from build123d import *

# Parameters (mm, degrees)
CYLINDER012_R               = 2
CYLINDER012_DEPTH           = 15
CYLINDER012_PLACEMENT_ANGLE = 1
CYLINDER013_R               = 2
CYLINDER013_DEPTH           = 15
CYLINDER006_R               = 9.75
CYLINDER006_DEPTH           = 6
CYLINDER004_R               = 31.5
CYLINDER004_DEPTH           = 3


with BuildPart() as cylinder012:
    # Cylinder012 → Cylinder012 (new body)
    with BuildSketch(Plane.XY):
        Circle(CYLINDER012_R)
    extrude(amount=CYLINDER012_DEPTH)


with BuildPart() as cylinder012_1:
    # Cylinder012 placement: moved
    add(cylinder012.part.moved(Location((0, -15, -1))).rotate(Axis((0, -15, -1), (0, 0, 1)), CYLINDER012_PLACEMENT_ANGLE))


with BuildPart() as fusion004:
    # Cylinder013 → Cylinder013 (new body)
    with BuildSketch(Plane(origin=(0, 15, -1), x_dir=(1, 0, 0), z_dir=(0, 0, 1))):
        Circle(CYLINDER013_R)
    extrude(amount=CYLINDER013_DEPTH)

    # Fusion004: union Cylinder012
    add(cylinder012_1.part)


with BuildPart() as cylinder006:
    # Cylinder006 → Cylinder006 (new body)
    with BuildSketch(Plane.XY):
        Circle(CYLINDER006_R)
    extrude(amount=CYLINDER006_DEPTH)


with BuildPart() as end_flange001:
    # Cylinder004 → Cylinder004 (new body)
    with BuildSketch(Plane.XY):
        Circle(CYLINDER004_R)
    extrude(amount=CYLINDER004_DEPTH)

    # Cut001: cut Cylinder006
    add(cylinder006.part, mode=Mode.SUBTRACT)

    # Cut009: cut Fusion004
    add(fusion004.part, mode=Mode.SUBTRACT)


with BuildPart() as end_flange001_1:
    # Cut009 placement: moved
    add(end_flange001.part.moved(Location((65, 0, 0))))


solid = end_flange001_1.part
Check sheet for the modelled part. Datum: model origin and axes. Units: mm. Give positions to 0.01 mm unless a question says otherwise; leave off trailing zeros. Loops run counter-clockwise (first coordinate to the right, second up) from the corner with the lowest first, then second, coordinate; pieces in that order, holes last. Notation, with made-up numbers: M 23,80.25 L 66,80.25 A27 ccw 66,110.25 Z; hole C 66,78.5 d2. An arc over 180 degrees is marked long. Return JSON: item names as keys, results as strings. Group by question number.
1. Mould release check, pull along Y, two halves, no side actions. Record for faces 1 (the flat face through (71.6, 7.4, 0)), 2 (the cylindrical face through (65, -13, 1)), 3 (the cylindrical face through (41.783, 21.289, 1.479)): released by +Y, released by -Y, zero draft, split by the parting line, or undercut.
2. Cross-section at A-A on y = 0. Record the boundary of the cut face in (x, z).
3. Thickness scan on L1, parallel to Y at x = 65, z = 1.35; L2, parallel to X at y = -15, z = 1.55; L3, parallel to X at y = -13.5, z = 1.8. Record the ranges inside material, lowest first.
4. Cross-section at B-B on x = 65. Record the boundary of the cut face in (y, z), plus the area to 4 significant figures.
5. Go/stop test with flat-tipped pins: pin 1 (1.5 mm diameter, centred on y = -20, z = 2, fed in from +X); pin 2 (5 mm diameter, centred on x = 65, y = 15, fed in from -Z); pin 3 (11.5 mm diameter, centred on x = 65, y = 0, fed in from -Z); pin 4 (1.5 mm diameter, centred on y = 6, z = 1.5, fed in from -X). Record where each tip stops, or that it passes through.
6. Cross-section at C-C on y = 15. Record the boundary of the cut face in (x, z).
7. Cross-section at D-D on z = 1.75. Record the boundary of the cut face in (x, y).
Return value:
{
 "1": {"face 1": "zero draft", "face 2": "undercut", "face 3": "split by the parting line"},
 "2": {"outline": "M 33.5,0 L 55.25,0 L 55.25,3 L 33.5,3 Z; M 74.75,0 L 96.5,0 L 96.5,3 L 74.75,3 Z"},
 "3": {"L1": "-31.5 to -17, -13 to -9.75, 9.75 to 13, 17 to 31.5", "L2": "37.3 to 63, 67 to 92.7", "L3": "36.54 to 63.68, 66.32 to 93.46"},
 "4": {"outline": "M -31.5,0 L -17,0 L -17,3 L -31.5,3 Z; M -13,0 L -9.75,0 L -9.75,3 L -13,3 Z; M 9.75,0 L 13,0 L 13,3 L 9.75,3 Z; M 17,0 L 31.5,0 L 31.5,3 L 17,3 Z", "area": "106.5 mm^2"},
 "5": {"pin 1": "x = 89.93", "pin 2": "z = 0", "pin 3": "through", "pin 4": "x = 33.94"},
 "6": {"outline": "M 37.3,0 L 63,0 L 63,3 L 37.3,3 Z; M 67,0 L 92.7,0 L 92.7,3 L 67,3 Z"},
 "7": {"outline": "C 65,0 d63; hole C 65,0 d19.5; hole C 65,-15 d4; hole C 65,15 d4"}
}
